Part model, mm, in its own coordinate system. Face numbers are marked on the shaded views. A direction names the side the tool comes from. Give positions to 0.01 mm unless a question says otherwise; leave off trailing zeros. Write each loop counter-clockwise with the first axis right and the second up, starting at its lowest first coordinate (ties: lowest second). Pieces come first, ordered by that corner, then holes. Notation, with made-up numbers: M 58.25,38.25 L 114.25,38.25 A25 cw 114.25,50.25 Z; hole C 2,50.25 d4. An arc over 180 degrees is marked long. Answer as CSV lines item,"result". Start each with the question number.
1) Tool access for the marked faces 4, 5, 6, 7 and 8: list every direction of +Z, -Z, +X, -X, +Y, -Y with a clear straight run to the whole face (end or side of a thin tool).
2) Slice it at B-B, the plane z = 7.75. Give the number of separate pieces and of enclosed holes in the cut face, plus the area to 3 significant figures.
3) Pin check, flat tips, straight feed: pin 1 Ø5 at (x, y) = (32.5, 10.5) entering from -Z; pin 2 Ø4 at (x, y) = (34.5, 27.5) entering from +Z; pin 3 Ø1.1 at (x, z) = (0.5, 7.5) entering from +Y. Stop position of each tip, or through.
4) Mould opens along X. For the marked faces 1, 2 and 3 say: pulls with the +X half, pulls with the -X half, needs draft (parallel to the pull), parting line crosses it, or undercut.
5) Slice it at C-C, the plane y = 4.6. Give the cut face in (x, z), plus the area to 3 significant figures.
6) Slice it at A-A, the plane x = 34.5. Give the cut face in (y, z), plus the area to 3 significant figures.
7) Wall check: line 1 along X through (y, z) = (27.65, -0.5); line 2 along X through (y, z) = (39, 1.5); line 3 along X through (y, z) = (31.5, 2.5). Give the ranges that are in metal, low to high. Write a range as from..to.
8) Slice it at D-D, the plane x = 66. Give the cut face in (y, z).
```python
from build123d import *

# Parameters (mm, degrees)
F1_DEPTH  = 2
F2_W      = 1
F2_H      = 7
F2_H_2    = 5.5
F2_W_2    = 5
F2_H_3    = 3
F2_W_3    = 4
F3_DEPTH  = 8
F4_W      = 68
F4_H      = 3
F4_W_2    = 1
F4_H_2    = 8.5
F5_DEPTH  = 1
F6_W      = 15
F6_H      = 10
F6_W_2    = 20
F7_DEPTH  = 5
F9_DEPTH  = 3.5
F10_R     = 3.5
F10_R_2   = 1.7
F11_DEPTH = 2
F13_R     = 2
F14_R     = 1


with BuildPart() as f1:
    # F0 (on Top) → F1 (new body)
    with BuildSketch(Plane.XY):
        Polygon((0, 7), (0, 0), (78, 0), (78, 33), (77, 33), (77, 38), (78, 38), (78, 42), (41, 42), (41, 41.1), (42, 41.1), (42, 39.9), (41, 39.9), (41, 27), (26, 27), (26, 39.9), (25, 39.9), (25, 41.1), (26, 41.1), (26, 42), (15, 42), (15, 41), (10, 41), (10, 42), (0, 42), (0, 35), (1, 35), (1, 30), (0, 30), (0, 12), (1, 12), (1, 7), align=None)
    extrude(amount=F1_DEPTH)

    # F2 (on face) → F3 (join)
    with BuildSketch(Plane.XY.offset(2)):
        Polygon((26, 42), (15, 42), (15, 41), (10, 41), (10, 42), (0, 42), (0, 35), (1, 35), (1, 39), (26, 39), (26, 39.9), (25, 39.9), (25, 41.1), (26, 41.1), align=None)
        with Locations((0.5, 26.5)):
            Rectangle(F2_W, F2_H)
        with Locations((0.5, 14.75)):
            Rectangle(F2_W, F2_H_2)
        Polygon((2, 7), (0, 7), (0, 0), (5, 0), (5, 3), (2, 3), align=None)
        Polygon((41, 39.9), (41, 39), (76, 39), (76, 30), (77, 30), (77, 25), (78, 25), (78, 33), (77, 33), (77, 38), (78, 38), (78, 42), (41, 42), (41, 41.1), (42, 41.1), (42, 39.9), align=None)
        Polygon((78, 0), (78, 16.5), (77, 16.5), (77, 3), (73, 3), (73, 0), align=None)
        with Locations((21, 1.5)):
            Rectangle(F2_W_2, F2_H_3)
        with Locations((39, 1.5)):
            Rectangle(F2_W_3, F2_H_3)
        with Locations((57, 1.5)):
            Rectangle(F2_W_2, F2_H_3)
    extrude(amount=F3_DEPTH)

    # F4 (on face) → F5 (join)
    with BuildSketch(Plane.XY.offset(2)):
        with Locations((39, 1.5)):
            Rectangle(F4_W, F4_H)
        with Locations((77.5, 20.75)):
            Rectangle(F4_W_2, F4_H_2)
    extrude(amount=F5_DEPTH)

    # F6 (on face) → F7 (join)
    with BuildSketch(Plane.XY.offset(2)):
        with Locations((12.5, 34)):
            Rectangle(F6_W, F6_H)
        with Locations((66, 34)):
            Rectangle(F6_W_2, F6_H)
    extrude(amount=F7_DEPTH)

    # F8 (on face) → F9 (join)
    with BuildSketch(Plane(origin=(0, 0, 0), x_dir=(1, 0, 0), z_dir=(0, 0, -1))):
        Polygon((78, 0), (0, 0), (0, -7), (1, -7), (1, -12), (0, -12), (0, -30), (1, -30), (1, -35), (0, -35), (0, -42), (10, -42), (10, -41), (15, -41), (15, -42), (26, -42), (26, -41.1), (25, -41.1), (25, -39.9), (26, -39.9), (26, -39), (2, -39), (2, -1), (77, -1), (77, -32), (76, -32), (76, -39), (41, -39), (41, -39.9), (42, -39.9), (42, -41.1), (41, -41.1), (41, -42), (78, -42), (78, -38), (77, -38), (77, -33), (78, -33), align=None)
    extrude(amount=F9_DEPTH)

    # F10 (on face) → F11 (join)
    with BuildSketch(Plane(origin=(0, 0, 0), x_dir=(1, 0, 0), z_dir=(0, 0, -1))):
        with Locations((73.25, -4.6)):
            Circle(F10_R)
        with Locations((73.25, -4.6)):
            Circle(F10_R_2, mode=Mode.SUBTRACT)
        with Locations((73.25, -27.65)):
            Circle(F10_R)
        with Locations((73.25, -27.65)):
            Circle(F10_R_2, mode=Mode.SUBTRACT)
        with Locations((15.25, -4.6)):
            Circle(F10_R)
        with Locations((15.25, -4.6)):
            Circle(F10_R_2, mode=Mode.SUBTRACT)
        with Locations((15.25, -27.65)):
            Circle(F10_R)
        with Locations((15.25, -27.65)):
            Circle(F10_R_2, mode=Mode.SUBTRACT)
    extrude(amount=F11_DEPTH)

    # F12: union 

    # F13
    f13_edges = [f1.edges().sort_by_distance(p)[0] for p in [
        (78, 0, 3.25),
        (78, 42, 3.25),
        (0, 0, 3.25),
        (0, 42, 3.25),
    ]]
    fillet(f13_edges, radius=F13_R)

    # F14
    f14_edges = [f1.edges().sort_by_distance(p)[0] for p in [
        (77, 1, -1.75),
    ]]
    fillet(f14_edges, radius=F14_R)


solid = f1.part
```
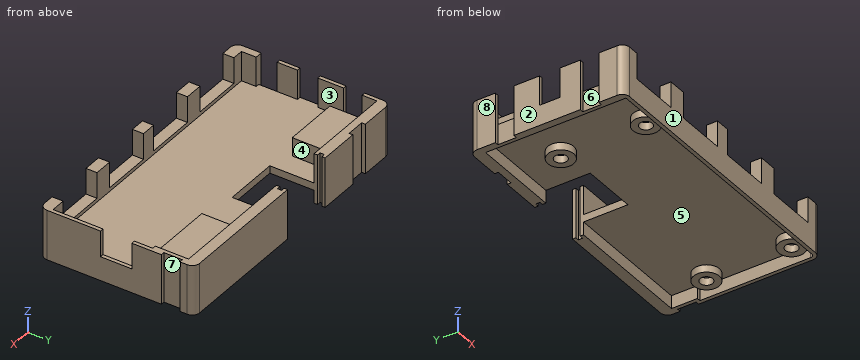
Found:
1,face 4,"+Z"
1,face 5,"-Z"
1,face 6,"+Z, -Z, -X"
1,face 7,"+Z, -Z, +X"
1,face 8,"+Z, -Z, -X, +Y, -Y"
2,separate pieces,"9"
2,enclosed holes,"0"
2,area,"306 mm²"
3,pin 1,"z = 0"
3,pin 2,"z = 2"
3,pin 3,"y = 41.76"
4,face 1,"needs draft"
4,face 2,"pulls with the -X half"
4,face 3,"undercut"
5,outline,"M 0,-3.5 L 2,-3.5 L 2,0 L 11.75,0 L 11.75,-2 L 13.55,-2 L 13.55,0 L 16.95,0 L 16.95,-2 L 18.75,-2 L 18.75,0 L 69.75,0 L 69.75,-2 L 71.55,-2 L 71.55,0 L 74.95,0 L 74.95,-2 L 76.75,-2 L 76.75,0 L 77,0 L 77,-3.5 L 78,-3.5 L 78,10 L 77,10 L 77,2 L 2,2 L 2,10 L 0,10 Z"
5,area,"205 mm²"
6,outline,"M 0,-3.5 L 1,-3.5 L 1,0 L 27,0 L 27,2 L 3,2 L 3,3 L 0,3 Z"
6,area,"60.5 mm²"
7,line 1,"0..2, 11.75..13.55, 16.95..18.75, 69.75..71.55, 74.95..76.75, 77..78"
7,line 2,"0..26, 41..78"
7,line 3,"5..20, 56..78"
8,outline,"M 0,-3.5 L 1,-3.5 L 1,0 L 39,0 L 39,-3.5 L 42,-3.5 L 42,10 L 39,10 L 39,7 L 29,7 L 29,2 L 3,2 L 3,3 L 0,3 Z"
